Could you check a few things on this model? Use its own coordinates, in mm. A direction names the side the tool comes from. Coordinates: 2 decimals unless noted, no trailing zeros. Order: outer loops, then holes, each group sorted by start corner. A loop starts at its lowest first (then second) coordinate and runs counter-clockwise, first axis right, second up. Notation, with made-up numbers: (86.25, -38.75) -> (118.25, -38.75) arc R13 ccw to (118.25, -32.75) -> close; hole circle Ø10 at (75, -36.75). An arc over 180 degrees is marked (long way). Use a Markdown table: item, result. Add a question column.
1) If we section it at D-D (y = 73.5): Write out the boundary of the cut face in (x, z), plus the area to 4 significant figures.
2) If we section it at A-A (y = 15.06): Write out the boundary of the cut face in (x, z) (3 decimals).
3) If I drill on L1, parallel to Y at x = 20.6, z = -15 (1 decimal); L2, parallel to Y at x = 25, z = -15 (3 decimals); L3, parallel to Z at x = 24.25, y = 6.56, over which ranges is the centre line in solid material (lowest first)? Write a range as [from, to].
4) Which directions (+Z, -Z, +X, -X, +Y, -Y) give clear straight access to the entire face, cutting with the end or side of a thin tool? Please do faces 1 (the flat face through (22.1, 21.5, -13)), 2 (the flat face through (15, 0, -3)), 3 (the flat face through (1.267, 134.806, -14.79)).
5) Thinking about a two-plate mould opening in Z: for faces 4 (the flat face through (10, 31.1, -15)), 5 (the cylindrical face through (14.865, 104.88, -14.79)), 6 (the flat face through (25, -8, -8.025)), which applies, +Z half, -Z half, draft (parallel to the pull), parting line (faces both ways), or undercut?
6) If we section it at C-C (z = -15): Give the number of separate pieces and of enclosed holes in the cut face, plus the area to 3 significant figures.
7) Will these pins go through, and if not, where does the flat tip stop? pin 1 Ø4 at (x, z) = (34.5, -9) entering from +Y; pin 2 Ø10 at (y, z) = (68, -24) entering from -X; pin 3 Ø5 at (y, z) = (43, -22.5) entering from +X; pin 4 Ø2.5 at (x, z) = (14, -27) entering from -Y.
8) If we section it at B-B (x = 6.5): Write out the boundary of the cut face in (y, z).
Autodesk Inventor part; units mm, degrees
ref_plane "YZ Plane" through (0, 0, 0) normal (1, 0, 0) x (0, 1, 0)
ref_plane "XZ Plane" through (0, 0, 0) normal (0, 1, 0) x (-1, 0, 0)
ref_plane "XY Plane" through (0, 0, 0) normal (0, 0, 1) x (1, 0, 0)
sketch "Sketch1" plane through (0, 0, 0) normal (0, 0, 1) x (1, 0, 0)
  line L0 (0, 0) -> (25, 0)
  line L1 (25, 0) -> (25, 40)
  line L2 (25, 40) -> (0, 40)
  line L3 (0, 40) -> (0, 0)
  dimension "d1" = 25
  dimension "d2" = 40
  dimension "d3" = 25
extrude "Extrusion1" add sketch "Sketch1" against normal blind 30
sketch "Sketch2" plane through (25, 0, 0) normal (1, 0, 0) x (0, 0, -1)
  line L0 (0, 0) -> (30, 0)
  circle A0 centre (15, 6.56) radius 2.46
extrude "Extrusion2" cut sketch "Sketch2" against normal blind 30
sketch "Sketch3" plane through (0, 0, 0) normal (-1, 0, 0) x (0, 0, 1)
  line L0 (0, 0) -> (-30, 0)
  line L1 (-25.05, 0) -> (-4.95, 0)
  line L2 (-4.95, 0) -> (-4.95, 33.12)
  line L3 (-4.95, 33.12) -> (-25.05, 33.12)
  line L4 (-25.05, 33.12) -> (-25.05, 0)
  dimension "d11" = 20.1
extrude "Extrusion3" cut sketch "Sketch3" against normal blind 20
sketch "Sketch4" plane through (0, 0, 0) normal (0, -1, 0) x (1, 0, 0)
  line L0 (20, -4.95) -> (20, -25.05)
  line L1 (20, -15) -> (25, -15)
  line L2 (25, 0) -> (25, -30)
  line L3 (20, -8.025) -> (25, -8.025)
  line L4 (25, -8.025) -> (25, -21.975)
  line L5 (25, -21.975) -> (20, -21.975)
  line L6 (20, -21.975) -> (20, -8.025)
  line L7 (20, -8.025) -> (25, -21.975) construction
  line L8 (25, -8.025) -> (20, -21.975) construction
  line L9 (25, -12.54) -> (25, -17.46)
  point P0 (0, 0)
  point P1 (22.5, -15)
  dimension "d14" = 13.95
extrude "Extrusion4" add sketch "Sketch4" along normal blind 15
sketch "Sketch5" plane through (20, 0, 0) normal (-1, 0, 0) x (0, 0, 1)
  circle A0 centre (-15, 6.56) radius 2.46
  circle A1 centre (-15, 6.56) radius 4.7025
  circle A2 centre (-15, 6.56) radius 2.46
  circle A3 centre (-15, 6.56) radius 2.46
  point P0 (0, 0)
  dimension "d17" = 9.405
extrude "Extrusion5" cut sketch "Sketch5" against normal blind 2.1
sketch "Sketch6" plane through (25, 0, 0) normal (1, 0, 0) x (0, 0, -1)
  circle A0 centre (15, 6.56) radius 4.7025
  line L0 (15, 6.56) -> (15, 23.56)
  circle A1 centre (15, 23.56) radius 2.46
  point P0 (0, 0)
  dimension "d20" = 17
  dimension "d21" = 4.92
extrude "Extrusion6" cut sketch "Sketch6" against normal blind 10 contours A1
sketch "Sketch7" plane through (20, 0, 0) normal (-1, 0, 0) x (0, 0, 1)
  circle A0 centre (-15, 23.56) radius 2.46
  circle A1 centre (-15, 23.56) radius 4.7025
  point P0 (0, 0)
  dimension "d24" = 9.405
extrude "Extrusion7" cut sketch "Sketch7" against normal blind 2.1
sketch "Sketch9" plane through (25, 0, 0) normal (1, 0, 0) x (0, 0, -1)
  circle A0 centre (15, 6.56) radius 2.46
  circle A1 centre (15, 6.56) radius 2.46
  circle A2 centre (15, 23.56) radius 2.46
  circle A3 centre (15, 23.56) radius 2.46
  line L0 (30, 40) -> (30, 0)
  line L1 (30, 0) -> (30, 40)
  line L2 (30, 40) -> (0, 40)
  line L3 (0, 40) -> (0, 0)
  line L4 (0, 0) -> (8.025, 0)
  line L5 (21.975, 0) -> (21.975, -15)
  line L6 (21.975, -15) -> (8.025, -15)
  line L7 (8.025, -15) -> (8.025, 0)
  line L8 (0, 0) -> (8.025, 0)
  line L9 (21.975, 0) -> (30, 0)
extrude "Extrusion8" add sketch "Sketch9" along normal blind 5
sketch "Sketch10" plane through (0, 40, 0) normal (0, 1, 0) x (1, 0, 0)
  line L0 (0, 30) -> (30, 30)
  line L1 (30, 0) -> (0, 0)
  line L2 (0, 30) -> (30, 30)
  line L3 (30, 30) -> (30, 0)
  line L4 (30, 0) -> (0, 0)
  line L5 (0, 0) -> (0, 30)
extrude "Extrusion9" add sketch "Sketch10" along normal blind 30
sketch "Sketch12" plane through (30, 0, 0) normal (1, 0, 0) x (0, 0, -1)
  circle A0 centre (15, 6.56) radius 2.46
  line L0 (15, 6.56) -> (15, 15.06)
  circle A1 centre (15, 15.06) radius 2.525
  point P0 (0, 0)
  dimension "d31" = 8.5
  dimension "d33" = 5.05
extrude "Extrusion10" cut sketch "Sketch12" against normal blind 30 contours A1
sketch "Sketch15" plane through (0, 0, -25.05) normal (-1, 0, 0) x (0, 0, 1)
  line L0 (0, 33.12) -> (20.1, 33.12)
  line L1 (20.1, 33.12) -> (20.1, 0)
  line L2 (0, 33.12) -> (20.1, 33.12)
  line L3 (20.1, 33.12) -> (20.1, 31.1)
  line L4 (20.1, 31.1) -> (0, 31.1)
  line L5 (0, 31.1) -> (0, 33.12)
  point P0 (25.05, 0)
  dimension "d57" = 2.02
extrude "Extrusion13" add sketch "Sketch15" against normal blind 20
sketch "Sketch17" plane through (0, 0, 0) normal (0, 0, 1) x (1, 0, 0)
  line L0 (0, 70) -> (30, 70)
  line L1 (30, 70) -> (50.0622, 90.0622)
  line L2 (30, 70) -> (80, 70) construction
  line L3 (11.9522, 97.2454) -> (0, 85.2932)
  line L4 (0, 70) -> (0, 85.2932)
  line L5 (0, 70) -> (0, 0)
  line L6 (0, 70) -> (30, 70)
  line L7 (10.923, 112.2849) -> (0, 120.567)
  line L8 (2.5, 134.067) -> (0, 135.567)
  line L9 (2.5, 134.067) -> (5, 128.067)
  line L10 (2.5, 122.067) -> (0, 120.567)
  line L11 (2.5, 122.067) -> (5, 128.067)
  line L12 (50.0622, 105.3553) -> (50.0622, 120.567)
  line L13 (50.0622, 105.3553) -> (50.0622, 90.0622)
  line L14 (0, 135.567) -> (30, 135.567)
  line L15 (30, 135.567) -> (50.0622, 120.567)
  arc A0 (11.9522, 97.2454) -> (10.923, 112.2849) centre (4.8811, 104.3165) ccw
  dimension "d61" = 45
  dimension "d62" = 32.0271
  dimension "d71" = 30
  dimension "d72" = 10
extrude "Extrusion14" add sketch "Sketch17" against normal blind 30
properties part number "rec_c_12mm_x_30mm"
Answer sheet:
| question | item | result |
|---|---|---|
| 1 | outline | (0, -30) -> (33.5, -30) -> (33.5, 0) -> (0, 0) -> close |
| 1 | area | 1,005 mm2 |
| 2 | outline | (0, -30) -> (30, -30) -> (30, -17.525) -> (20, -17.525) -> (20, -25.05) -> (0, -25.05) -> close; (0, -4.95) -> (20, -4.95) -> (20, -12.475) -> (30, -12.475) -> (30, 0) -> (0, 0) -> close |
| 3 | L1 | [-15, 1.9], [11.3, 12.5], [17.6, 18.9], [28.3, 135.6] |
| 3 | L2 | [-15, 4.1], [9.02, 12.535], [17.585, 21.1], [26.02, 135.567] |
| 3 | L3 | [-30, -17.46], [-12.54, 0] |
| 4 | face 1 | -X |
| 4 | face 2 | +Z, +X, -X, -Y |
| 4 | face 3 | +Z, -Z, -X |
| 5 | face 4 | undercut |
| 5 | face 5 | draft |
| 5 | face 6 | +Z half |
| 6 | separate pieces | 4 |
| 6 | enclosed holes | 0 |
| 6 | area | 4,020 mm2 |
| 7 | pin 1 | y = 133.7 |
| 7 | pin 2 | x = 0 |
| 7 | pin 3 | x = 30 |
| 7 | pin 4 | y = 0 |
| 8 | outline | (0, -30) -> (91.79, -30) -> (91.79, 0) -> (0, 0) -> (0, -4.95) -> (31.1, -4.95) -> (31.1, -25.05) -> (0, -25.05) -> close; (115.64, -30) -> (135.57, -30) -> (135.57, 0) -> (115.64, 0) -> close |
